Design review of the part built by this model. Coordinates are the model's own, in mm. Face numbers are marked on the shaded views. A direction names the side the tool comes from. Give positions to 0.01 mm unless a question says otherwise; leave off trailing zeros. Write each loop counter-clockwise with the first axis right and the second up, starting at its lowest first coordinate (ties: lowest second). Pieces come first, ordered by that corner, then holes.
```python
from build123d import *

# Parameters (mm, degrees)
F1_DEPTH = 2
F3_DEPTH = 10
F5_DEPTH = 1
F6_DEPTH = 0.5
F7_R     = 1


with BuildPart() as f1:
    # F0 (on Top) → F1 (new body)
    with BuildSketch(Plane.XY):
        with BuildLine():
            Line((-2.078642603, 0), (47.9039736092, 2.6289783418))
            ThreePointArc((47.9039736092, 2.6289783418), (32.9834717321, 36.2761769642), (0, 52.6115968823))
            Line((0, 52.6115968823), (-25.8684456348, 21.8530613929))
            Line((-25.8684456348, 21.8530613929), (-2.078642603, 0))
        make_face()
    extrude(amount=F1_DEPTH)

    # F2 (on face) → F3 (join)
    with BuildSketch(Plane.XY.offset(2)):
        Polygon((-3.4849730935, 31.2140034176), (-4.5563918538, 28.3914133906), (20.8157394081, 6.5072686411), (22.6687969397, 8.6556742318), align=None)
    extrude(amount=F3_DEPTH)

    # F4 (on face) → F5 (cut)
    with BuildSketch(Plane.XY.offset(2)):
        Polygon((-2.078642603, 0), (2.9054336124, 0.2621517123), (-18.4005183491, 30.7327022377), (-25.8684456348, 21.8530613929), align=None)
    extrude(amount=-F5_DEPTH, mode=Mode.SUBTRACT)

    # F6 (cut): a face of the model
    f6_faces = [f1.faces().sort_by_distance(p)[0] for p in [
        (-12.6099622949, 15.3981218479, 1),
    ]]
    extrude(f6_faces, amount=-F6_DEPTH, mode=Mode.SUBTRACT)

    # F7
    f7_edges = [f1.edges().sort_by_distance(p)[0] for p in [
        (-7.747542, 15.497427, 0.5),
    ]]
    fillet(f7_edges, radius=F7_R)


solid = f1.part
```
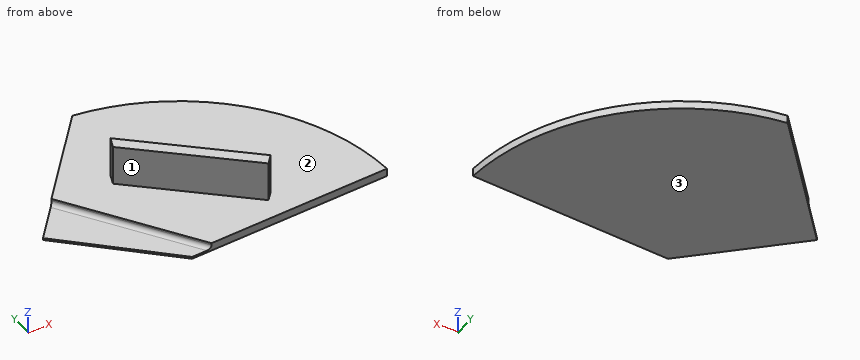
(1) Consider section B-B, the plane z = 7.75. Give the boundary of the cut face in (x, y).
Resolved:
outline: (-4.56, 28.39) - (20.82, 6.51) - (22.67, 8.66) - (-3.48, 31.21) - close
(2) To check wall thickness, follow L1, parallel to Z at x = -20.5, y = 27; L2, parallel to Z at x = 10, y = 29; L3, parallel to X at y = 27, z = 7.25. State the ranges of each line that lie inside material, in increasing order.
Resolved:
L1: z = 0 to 0.5
L2: z = 0 to 2
L3: x = -2.94 to 1.4
(3) Consider section C-C, the plane y = 36. Give the boundary of the cut face in (x, z), then the cut area to 3 significant figures.
Resolved:
outline: (-13.97, 0) - (33.25, 0) - (33.25, 2) - (-13.97, 2) - close
area: 94.4 mm2
(4) Clearance check with flat-ended pins moving along their axes: P1, Ø6, axis at y = 37.5, z = 5.5, coming from the +X side; P2, Ø1, axis at x = -7, y = 6, coming from the +Z side; P3, Ø22, axis at x = -17.5, y = 13, coming from the +Z side; P4, Ø2, axis at y = 25.5, z = 4.5, coming from the +X side. State where each tip first meets the part, or that it passes through.
Resolved:
P1: passes through
P2: stops at z = 0.5
P3: stops at z = 2
P4: stops at x = 4.3
(5) Tool access review of the marked faces 1, 2 and 3: name each direction out of +Z, -Z, +X, -X, +Y, -Y from which nothing blocks a thin tool from reaching the whole face with its end or side.
Resolved:
face 1: +Z, -X, -Y
face 2: +Z
face 3: -Z, +X, -X, +Y, -Y
(6) Consider section A-A, the plane x = 6.5. Give the boundary of the cut face in (y, z).
Resolved:
outline: (0.45, 0) - (51.47, 0) - (51.47, 2) - (22.6, 2) - (22.6, 12) - (18.85, 12) - (18.85, 2) - (0.45, 2) - close
